Source: CAD feature listing. Evaluate the final solid. Frame: model axes, mm. A direction names the side the tool comes from. Round coordinates to 2 decimals unless told otherwise and drop trailing zeros. Loops run counter-clockwise (first coordinate to the right, second up) from the corner with the lowest first, then second, coordinate; pieces in that order, holes last. Notation, with made-up numbers: (-39.75, -20.5) - (-5.75, -20.5) arc R31 ccw to (-5.75, 14.5) - close; hole circle Ø9 at (-2.75, -28.5). An arc over 180 degrees is marked (long way). One line per question, with ' | ' between items.
from build123d import *

# Parameters (mm, degrees)
F1_DEPTH = 2.35
F2_R     = 4.25
F2_R_2   = 2.75
F3_DEPTH = 3.5
F4_R     = 1.5
F4_R_2   = 1
F5_DEPTH = 25
F6_R     = 4.5
F6_R_2   = 3.5
F6_R_3   = 3
F6_R_4   = 1.5
F7_DEPTH = 1


with BuildPart() as f1:
    # F0 (on Top) → F1 (new body)
    with BuildSketch(Plane.XY):
        with BuildLine():
            Line((-16.890331, -2.46934), (-4.043822, -4.5))
            ThreePointArc((-4.043822, -4.5), (0, -6.05), (4.043822, -4.5))
            Line((4.043822, -4.5), (16.890331, -2.46934))
            ThreePointArc((16.890331, -2.46934), (19, 0), (16.890331, 2.46934))
            Line((16.890331, 2.46934), (4.043822, 4.5))
            ThreePointArc((4.043822, 4.5), (0, 6.05), (-4.043822, 4.5))
            Line((-4.043822, 4.5), (-16.890331, 2.46934))
            ThreePointArc((-16.890331, 2.46934), (-19, 0), (-16.890331, -2.46934))
        make_face()
    extrude(amount=F1_DEPTH)

    # F2 (on face) → F3 (join)
    with BuildSketch(Plane(origin=(0, 0, 0), x_dir=(1, 0, 0), z_dir=(0, 0, -1))):
        Circle(F2_R)
        Circle(F2_R_2, mode=Mode.SUBTRACT)
    extrude(amount=F3_DEPTH)

    # F4 (on face) → F5 (cut)
    with BuildSketch(Plane(origin=(0, 0, 0), x_dir=(1, 0, 0), z_dir=(0, 0, -1))):
        Circle(F4_R)
        with Locations((-7.5, 0)):
            Circle(F4_R_2)
        with Locations((-10.5, 0)):
            Circle(F4_R_2)
        with Locations((-13.5, 0)):
            Circle(F4_R_2)
        with Locations((-16.5, 0)):
            Circle(F4_R_2)
        with Locations((7.5, 0)):
            Circle(F4_R_2)
        with Locations((10.5, 0)):
            Circle(F4_R_2)
        with Locations((13.5, 0)):
            Circle(F4_R_2)
        with Locations((16.5, 0)):
            Circle(F4_R_2)
    extrude(amount=-F5_DEPTH, mode=Mode.SUBTRACT)

    # F6 (on face) → F7 (cut)
    with BuildSketch(Plane.XY.offset(2.35)):
        Circle(F6_R)
        Circle(F6_R_2, mode=Mode.SUBTRACT)
        Circle(F6_R_3)
        Circle(F6_R_4, mode=Mode.SUBTRACT)
    extrude(amount=-F7_DEPTH, mode=Mode.SUBTRACT)


solid = f1.part
1. Material intervals for probe 1 along Y at (x, z) = (0, -1.6); probe 2 along X at (y, z) = (1.25, 1.65); probe 3 along X at (y, z) = (-2, -0.65), sorted ascending.
Worked out:
probe 1: y = -4.25 to -2.75, 2.75 to 4.25 | probe 2: x = -18.67 to -4.32, -3.27 to -2.73, 2.73 to 3.27, 4.32 to 18.67 | probe 3: x = -3.75 to -1.89, 1.89 to 3.75
2. Section query B-B, the plane z = 0.65. Give the number of separate pieces and of enclosed holes in the cut face, plus the area to 3 significant figures.
Worked out:
separate pieces: 1 | enclosed holes: 9 | area: 253 mm2
3. Contact query for flat-ended pins moving along their axis: P1, Ø2, axis at x = 11, y = 4.5, coming from the +Z side; P2, Ø1.5, axis at x = 15, z = -0.5, coming from the +Y side; P3, Ø2, axis at y = -1, z = -1.5, coming from the +X side; P4, Ø1, axis at y = -3, z = -1.5, coming from the +X side. Output: stop coordinate, or through.
Worked out:
P1: passes through | P2: stops at y = 2.86 | P3: stops at x = 4.25 | P4: stops at x = 3.44
4. Access query for faces 1 (the cylindrical face through (2.285, -3.584, -1.726)), 2 (the cylindrical face through (3.233, -1.341, 1.857)), 3 (the cylindrical face through (-19, 0, 1)). Directions: +Z, -Z, +X, -X, +Y, -Y. A direction counts if a zero-diameter tool reaches every point of the face in a straight line with its end or side. Return the directions, or none.
Worked out:
face 1: -Z | face 2: +Z | face 3: +Z, -Z, -X
5. Mould query, pull axis Y, two halves, no side actions, for faces 4 (the cylindrical face through (0.06, 6.05, 1.16)), 5 (the cylindrical face through (19, 0, 1)), 6 (the cylindrical face through (6.7, 0.6, 1.2)), 7 (the flat face through (10.38, -3.5, 1.16)). Classes: released by +Y, released by -Y, zero draft, split by the parting line, or undercut.
Worked out:
face 4: released by +Y | face 5: split by the parting line | face 6: undercut | face 7: released by -Y
6. Section query A-A, the plane x = 0. Return loops of the section in (y, z), plus the area to 3 significant figures.
Worked out:
outline: (-6.05, 0) - (-4.25, 0) - (-4.25, -3.5) - (-2.75, -3.5) - (-2.75, 0) - (-1.5, 0) - (-1.5, 1.35) - (-3, 1.35) - (-3, 2.35) - (-3.5, 2.35) - (-3.5, 1.35) - (-4.5, 1.35) - (-4.5, 2.35) - (-6.05, 2.35) - close; (1.5, 0) - (2.75, 0) - (2.75, -3.5) - (4.25, -3.5) - (4.25, 0) - (6.05, 0) - (6.05, 2.35) - (4.5, 2.35) - (4.5, 1.35) - (3.5, 1.35) - (3.5, 2.35) - (3, 2.35) - (3, 1.35) - (1.5, 1.35) - close | area: 26.9 mm2
7. Section query D-D, the plane x = 8. Return loops of the section in (y, z), plus the area to 3 significant figures.
Worked out:
outline: (-3.87, 0) - (-0.87, 0) - (-0.87, 2.35) - (-3.87, 2.35) - close; (0.87, 0) - (3.87, 0) - (3.87, 2.35) - (0.87, 2.35) - close | area: 14.1 mm2
